Autodesk Inventor part; units mm, degrees
ref_plane "YZ Plane" through (0, 0, 0) normal (1, 0, 0) x (0, 1, 0)
ref_plane "XZ Plane" through (0, 0, 0) normal (0, 1, 0) x (-1, 0, 0)
ref_plane "XY Plane" through (0, 0, 0) normal (0, 0, 1) x (1, 0, 0)
sketch "Sketch1" plane through (0, 0, 0) normal (0, 0, 1) x (1, 0, 0)
  line L0 (5, 2.8868) -> (5, -2.8868)
  line L1 (5, -2.8868) -> (0, -5.7735)
  line L2 (0, -5.7735) -> (-5, -2.8868)
  line L3 (-5, -2.8868) -> (-5, 2.8868)
  line L4 (-5, 2.8868) -> (0, 5.7735)
  line L5 (0, 5.7735) -> (5, 2.8868)
  point P0 (0, 0)
  point P1 (0, 0)
  dimension "d0" = 10
extrude "Extrusion1" add sketch "Sketch1" along normal blind 7
sketch "Sketch2" plane through (0, 0, 7) normal (0, 0, 1) x (1, 0, 0)
  circle A0 centre (0, 0) radius 3
  dimension "d3" = 6
extrude "Extrusion2" add sketch "Sketch2" along normal blind 5
fillet "Fillet1" radius 1 6 edges at (-5, 2.8868, 3.5) (-5, -2.8868, 3.5) (0, -5.7735, 3.5) (5, -2.8868, 3.5) (5, 2.8868, 3.5) (0, 5.7735, 3.5)
chamfer "Chamfer1" distance 0.5 angle 45 1 edges at (-3, 0, 7)
chamfer "Chamfer2" distance 0.5 angle 45 25 edges at (-3, 0, 12) (2.5, -4.3301, 7) (4.866, -2.8094, 7) (5, 0, 7) (4.866, 2.8094, 7) (2.5, 4.3301, 7) (0, 5.6188, 7) (-2.5, 4.3301, 7) (-4.866, 2.8094, 7) (-5, 0, 7) (-4.866, -2.8094, 7) (-2.5, -4.3301, 7) (0, -5.6188, 7) (2.5, -4.3301, 0) (4.866, -2.8094, 0) (5, 0, 0) (4.866, 2.8094, 0) (2.5, 4.3301, 0) (0, 5.6188, 0) (-2.5, 4.3301, 0) (-4.866, 2.8094, 0) (-5, 0, 0) (-4.866, -2.8094, 0) (-2.5, -4.3301, 0) (0, -5.6188, 0)
properties part number "TPU-legs" material "Rubber"
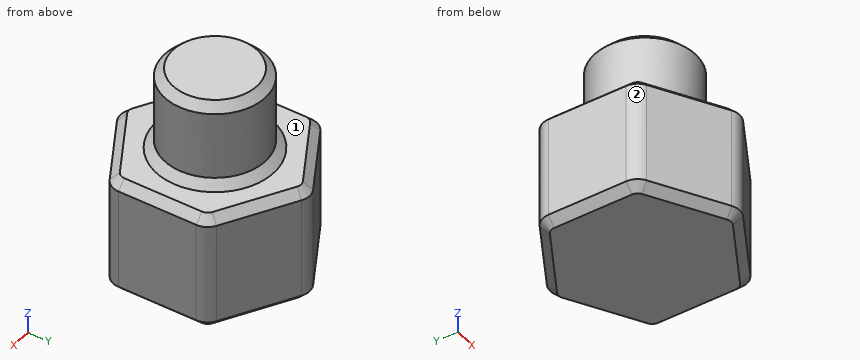
Model file for the job. Use its own axes, mm. Face numbers are marked on the shaded views. A direction names the side the tool comes from. Coordinates: 2 decimals unless noted, no trailing zeros. Order: outer loops, then holes, each group sorted by start corner. A loop starts at its lowest first (then second) coordinate and runs counter-clockwise, first axis right, second up. Notation, with made-up numbers: M 0,15.25 L 17,15.25 A10 cw 17,21.25 Z; hole C 9.5,32.5 d4. An arc over 180 degrees is marked long. Answer as CSV lines item,"result".
(1) Wall check: line 1 along Z through (x, y) = (3.5, 0.75); line 2 along Y through (x, z) = (-4.5, 3.25); line 3 along Y through (x, z) = (-0.5, 4). Give the ranges that are in metal, low to high.
Geometry says:
line 1,"z = 0 to 7"
line 2,"y = -3.18 to 3.18"
line 3,"y = -5.48 to 5.48"
(2) Band-saw the part on C-C, the plane x = 0. List the corners of the cut face in (y, z), then the cut area to 3 significant figures.
Geometry says:
outline,"M -5.62,0.5 L -5.12,0 L 5.12,0 L 5.62,0.5 L 5.62,6.5 L 5.12,7 L 3.5,7 L 3,7.5 L 3,11.5 L 2.5,12 L -2.5,12 L -3,11.5 L -3,7.5 L -3.5,7 L -5.12,7 L -5.62,6.5 Z"
area,"108 mm2"
(3) Band-saw the part on D-D, the plane z = 7.75. List the corners of the cut face in (x, y), then the cut area to 3 significant figures.
Geometry says:
outline,"C 0,0 d6"
area,"28.3 mm2"
(4) Band-saw the part on A-A, the plane y = 0. List the corners of the cut face in (x, z).
Geometry says:
outline,"M -5,0.5 L -4.5,0 L 4.5,0 L 5,0.5 L 5,6.5 L 4.5,7 L 3.5,7 L 3,7.5 L 3,11.5 L 2.5,12 L -2.5,12 L -3,11.5 L -3,7.5 L -3.5,7 L -4.5,7 L -5,6.5 Z"
(5) 3-axis set-ups, long thin cutter, end or side, ignore diameter. For the marked faces 1 and 2: which of +Z, -Z, +X, -X, +Y, -Y reach the whole face in a straight line?
Geometry says:
face 1,"+Z"
face 2,"+Z, -Z, -X, -Y"
(6) Band-saw the part on B-B, the plane z = 1.75. List the corners of the cut face in (x, y).
Geometry says:
outline,"M -5,-2.31 A1 ccw -4.5,-3.18 L -0.5,-5.48 A1 ccw 0.5,-5.48 L 4.5,-3.18 A1 ccw 5,-2.31 L 5,2.31 A1 ccw 4.5,3.18 L 0.5,5.48 A1 ccw -0.5,5.48 L -4.5,3.18 A1 ccw -5,2.31 Z"
(7) Flat gauge pins, fed straight in: pin 1 (5 mm diameter, centred on x = 3.5, z = 8.5, fed in from +Y); pin 2 (3 mm diameter, centred on x = -1.5, y = -3, fed in from -Z); pin 3 (3 mm diameter, centred on y = -4, z = 6, fed in from -X); pin 4 (1.5 mm diameter, centred on x = -3.5, z = 6.5, fed in from +Y). Where does each tip first touch, or does it go through?
Geometry says:
pin 1,"stops at y = 4.62"
pin 2,"stops at z = 0"
pin 3,"stops at x = -4.98"
pin 4,"stops at y = 4.19"
